```python
from build123d import *

# Parameters (mm, degrees)
CUT_EXTRUDE_1_DEPTH = 3
CUT_EXTRUDE_2_DEPTH = 3.5
CHAMFER_1_SIZE      = 1


with BuildPart() as part:
    # 草图1 → 旋转1 (revolve)
    with BuildSketch(Plane.XY, mode=Mode.PRIVATE) as revolve_1_sk:
        Polygon((0, 0), (0, 7.5), (28, 7.5), (28, 8.5), (49, 8.5), (49, 7.5), (51, 7.5), (51, 5), (56, 5), (56, 15), (61, 15), (61, 10), (63, 10), (63, 11), (94, 11), (94, 9), (96, 9), (96, 10), (110, 10), (110, 8.5), (141, 8.5), (141, 7), (143, 7), (143, 7.5), (155, 7.5), (155, 0), align=None)
    revolve(revolve_1_sk.sketch.rotate(Axis((0, 0, 0), (1, 0, 0)), 90), axis=Axis((0, 0, 0), (1, 0, 0)))

    # 草图2 → 切除-拉伸1 (cut)
    with BuildSketch(Plane.XY.offset(7.5)):
        with BuildLine():
            Line((18, -2.5), (7, -2.5))
            ThreePointArc((7, -2.5), (4.5, 0), (7, 2.5))
            Line((7, 2.5), (18, 2.5))
            ThreePointArc((18, 2.5), (20.5, 0), (18, -2.5))
        make_face()
    extrude(amount=-CUT_EXTRUDE_1_DEPTH, mode=Mode.SUBTRACT)

    # 草图3 → 切除-拉伸2 (cut)
    with BuildSketch(Plane(origin=(0, 0, 11), x_dir=(-1, 0, 0), z_dir=(0, 0, 1))):
        with BuildLine():
            Line((-88, 3), (-69, 3))
            ThreePointArc((-69, 3), (-66, 0), (-69, -3))
            Line((-69, -3), (-88, -3))
            ThreePointArc((-88, -3), (-91, 0), (-88, 3))
        make_face()
    extrude(amount=-CUT_EXTRUDE_2_DEPTH, mode=Mode.SUBTRACT)

    # 倒角1
    chamfer_1_edges = [part.edges().sort_by_distance(p)[0] for p in [
        (155, 0, -7.5),
        (110, 0, -10),
        (0, 0, -7.5),
    ]]
    chamfer(chamfer_1_edges, length=CHAMFER_1_SIZE)


solid = part.part
```
Here's how the part is built. I have some questions about the finished solid (model axes, mm). A direction names the side the tool comes from. Coordinates: 2 decimals unless noted, no trailing zeros. Order: outer loops, then holes, each group sorted by start corner. A loop starts at its lowest first (then second) coordinate and runs counter-clockwise, first axis right, second up. Notation, with made-up numbers: (86.25, 4.5) - (110.25, 4.5) arc R12 ccw to (110.25, 20.5) - close; hole circle Ø4 at (-18, 59.25). An arc over 180 degrees is marked (long way). One line per question, with ' | ' between items. Start each with the question number.
1. I'm going to push flat-ended pins straight in: pin 1 Ø5.5 at (x, y) = (11.5, 0) entering from +Z; pin 2 Ø2 at (x, z) = (10, 6.5) entering from +Y; pin 3 Ø2 at (y, z) = (-8, 8.5) entering from +X. Where does each tip first touch, or does it pass through?
2. Which directions (+Z, -Z, +X, -X, +Y, -Y) give clear straight access to the entire face, cutting with the end or side of a thin tool? Please do faces 1 (the cylindrical face through (4.5, -0.1, 6)), 2 (the cylindrical face through (142.01, 6.21, 3.23)), 3 (the cylindrical face through (148.577, -6.324, 4.032)).
3. If we section it at A-A (x = 115): Write out the boundary of the cut face in (y, z).
4. If we section it at B-B (x = 79): Write out the boundary of the cut face in (y, z).
5. Please list where these lines run through material, in increasing order: line 1 along X through (y, z) = (9, -5); line 2 along Y through (x, z) = (64.5, 8.5); line 3 along X through (y, z) = (13.75, 5.5). Write a range as [from, to].
Model answer:
1) pin 1: stops at z = 7.07 | pin 2: stops at y = 5.1 | pin 3: stops at x = 94
2) face 1: +Z | face 2: none | face 3: +X
3) outline: circle Ø17 at (0, 0)
4) outline: (-3, 7.5) - (-3, 10.58) arc R11 ccw (long way) to (3, 10.58) - (3, 7.5) - close
5) line 1: x = [56, 61], [63, 94] | line 2: y = [-6.98, 6.98] | line 3: x = [56, 61]
